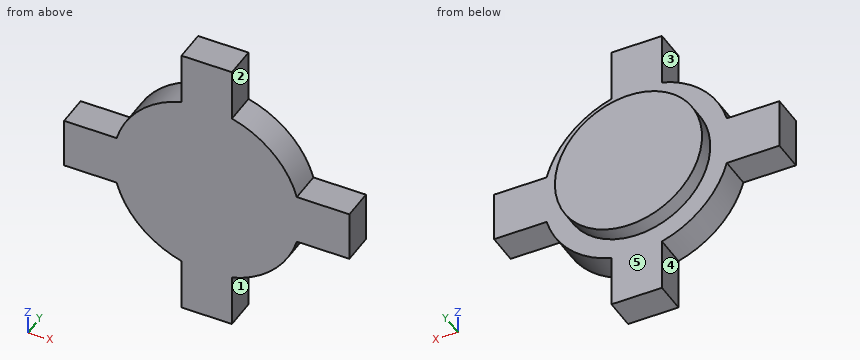
from build123d import *

# Parameters (mm, degrees)
EXTRUDE_1_DEPTH = 3
SKETCH_2_R      = 7
EXTRUDE_2_DEPTH = 1.5


with BuildPart() as part:
    # 草图1 → 凸台-拉伸1 (new body)
    with BuildSketch(Plane(origin=(0, 0, 0), x_dir=(1, 0, 0), z_dir=(0, 1, 0))):
        with BuildLine():
            Line((-13.570297544, 2.4), (-8.570297544, 2.4))
            ThreePointArc((-8.570297544, 2.4), (-6.293250353, 6.293250353), (-2.4, 8.570297544))
            Line((-2.4, 8.570297544), (-2.4, 13.570297544))
            Line((-2.4, 13.570297544), (2.4, 13.570297544))
            Line((2.4, 13.570297544), (2.4, 8.570297544))
            ThreePointArc((2.4, 8.570297544), (6.293250353, 6.293250353), (8.570297544, 2.4))
            Line((8.570297544, 2.4), (13.570297544, 2.4))
            Line((13.570297544, 2.4), (13.570297544, -2.4))
            Line((13.570297544, -2.4), (8.570297544, -2.4))
            ThreePointArc((8.570297544, -2.4), (6.293250353, -6.293250353), (2.4, -8.570297544))
            Line((2.4, -8.570297544), (2.4, -13.570297544))
            Line((2.4, -13.570297544), (-2.4, -13.570297544))
            Line((-2.4, -13.570297544), (-2.4, -8.570297544))
            ThreePointArc((-2.4, -8.570297544), (-6.293250353, -6.293250353), (-8.570297544, -2.4))
            Line((-8.570297544, -2.4), (-13.570297544, -2.4))
            Line((-13.570297544, -2.4), (-13.570297544, 2.4))
        make_face()
    extrude(amount=EXTRUDE_1_DEPTH)

    # 草图2 → 凸台-拉伸2 (add)
    with BuildSketch(Plane(origin=(0, 3, 0), x_dir=(1, 0, 0), z_dir=(0, 1, 0))):
        Circle(SKETCH_2_R)
    extrude(amount=EXTRUDE_2_DEPTH)


solid = part.part
The listing builds one solid part. Answer for the finished solid, in the listing's coordinates (mm). Face numbers are marked on the shaded views. A direction names the side the tool comes from. Coordinates: 2 decimals unless noted, no trailing zeros. Order: outer loops, then holes, each group sorted by start corner. A loop starts at its lowest first (then second) coordinate and runs counter-clockwise, first axis right, second up. Notation, with made-up numbers: (42.25, 62) -> (88.25, 62) arc R29 cw to (88.25, 99) -> close; hole circle Ø5 at (4, 41.5). An arc over 180 degrees is marked (long way). Answer in a Markdown table with one row per item. Add a question column.
Item 1: Find the intervals of material crossed by L1, parallel to X at y = 2.65, z = -12.5; L2, parallel to X at y = 3.2, z = 0, in increasing order. Write a range as from..to.
Item 2: Which of the six approach directions +Z, -Z, +X, -X, +Y, -Y give full straight-line access (tool end or side, diameter ignored) to the marked faces 1, 2, 3, 4 and 5?
Item 3: Each of these flat-tipped pins is pushed along its axis until it touches: P1, Ø0.9, axis at x = 12, y = 1, coming from the -Z side; P2, Ø2.5, axis at y = 1.5, z = -10, coming from the +X side; P3, Ø2.5, axis at y = 1, z = 12, coming from the -X side; P4, Ø5, axis at x = -9.5, z = -8.5, coming from the -Y side. Where does it stop, or does it pass through?
Item 4: Find section B-B (z = 0). Write down the section's boundary in (x, y).
Item 5: Find section D-D (x = -10.5). Write down the section's boundary in (y, z).
Item 6: Find section A-A (y = 0.8). Write down the section's boundary in (x, z), then the cut area to 3 significant figures.
Item 7: Find section C-C (x = 0). Write down the section's boundary in (y, z).
Result set:
| question | item | result |
|---|---|---|
| 1 | L1 | x = -2.4..2.4 |
| 1 | L2 | x = -7..7 |
| 2 | face 1 | -Z, +X, +Y, -Y |
| 2 | face 2 | +Z, +X, +Y, -Y |
| 2 | face 3 | +Z, -X, +Y, -Y |
| 2 | face 4 | -Z, -X, +Y, -Y |
| 2 | face 5 | +Y |
| 3 | P1 | stops at z = -2.4 |
| 3 | P2 | stops at x = 2.4 |
| 3 | P3 | stops at x = -2.4 |
| 3 | P4 | passes through |
| 4 | outline | (-13.57, 0) -> (13.57, 0) -> (13.57, 3) -> (7, 3) -> (7, 4.5) -> (-7, 4.5) -> (-7, 3) -> (-13.57, 3) -> close |
| 5 | outline | (0, -2.4) -> (3, -2.4) -> (3, 2.4) -> (0, 2.4) -> close |
| 6 | outline | (-13.57, -2.4) -> (-8.57, -2.4) arc R8.9 ccw to (-2.4, -8.57) -> (-2.4, -13.57) -> (2.4, -13.57) -> (2.4, -8.57) arc R8.9 ccw to (8.57, -2.4) -> (13.57, -2.4) -> (13.57, 2.4) -> (8.57, 2.4) arc R8.9 ccw to (2.4, 8.57) -> (2.4, 13.57) -> (-2.4, 13.57) -> (-2.4, 8.57) arc R8.9 ccw to (-8.57, 2.4) -> (-13.57, 2.4) -> close |
| 6 | area | 341 mm² |
| 7 | outline | (0, -13.57) -> (3, -13.57) -> (3, -7) -> (4.5, -7) -> (4.5, 7) -> (3, 7) -> (3, 13.57) -> (0, 13.57) -> close |
